from build123d import *

# Parameters (mm, degrees)
SKETCH_1_W          = 12
SKETCH_1_H          = 12
EXTRUDE_1_DEPTH     = 9.5
SKETCH_2_R          = 5.5
EXTRUDE_2_DEPTH     = 455
SKETCH_3_W          = 12
SKETCH_3_H          = 12
EXTRUDE_3_DEPTH     = 12.5
SKETCH_4_R          = 4
EXTRUDE_4_DEPTH     = 8
CUT_EXTRUDE_START   = -6
SKETCH_6_R          = 2.5
CUT_EXTRUDE_2_DEPTH = 6
FILLET_1_R          = 2
SKETCH_7_R          = 4
EXTRUDE_5_DEPTH     = 8


with BuildPart() as part:
    # 草图1 → 凸台-拉伸1 (new body)
    with BuildSketch(Plane.XY):
        Rectangle(SKETCH_1_W, SKETCH_1_H)
    extrude(amount=EXTRUDE_1_DEPTH)

    # 草图2 → 凸台-拉伸2 (add)
    with BuildSketch(Plane.XY.offset(9.5)):
        Circle(SKETCH_2_R)
    extrude(amount=EXTRUDE_2_DEPTH)

    # 草图3 → 凸台-拉伸3 (add)
    with BuildSketch(Plane.XY.offset(464.5)):
        Rectangle(SKETCH_3_W, SKETCH_3_H)
    extrude(amount=EXTRUDE_3_DEPTH)

    # 草图4 → 凸台-拉伸4 (add)
    with BuildSketch(Plane.XY.offset(477)):
        Circle(SKETCH_4_R)
    extrude(amount=EXTRUDE_4_DEPTH)

    # 草图6 → 切除-拉伸2 (cut)
    with BuildSketch(Plane(origin=(0, 6, 0), x_dir=(1, 0, 0), z_dir=(0, 1, 0)).offset(CUT_EXTRUDE_START)):
        with Locations((0, -4.75)):
            Circle(SKETCH_6_R)
        with Locations((0, -469.25)):
            Circle(SKETCH_6_R)
    extrude(amount=CUT_EXTRUDE_2_DEPTH, mode=Mode.SUBTRACT)

    # 圆角1
    fillet_1_edges = [part.edges().sort_by_distance(p)[0] for p in [
        (6, -6, 470.75),
        (6, 6, 470.75),
        (-6, 6, 470.75),
        (-6, -6, 470.75),
        (6, -6, 4.75),
        (-6, -6, 4.75),
        (-6, 6, 4.75),
        (6, 6, 4.75),
    ]]
    fillet(fillet_1_edges, radius=FILLET_1_R)

    # 草图7 → 凸台-拉伸5 (add)
    with BuildSketch(Plane(origin=(0, 0, 0), x_dir=(-1, 0, 0), z_dir=(0, 0, -1))):
        Circle(SKETCH_7_R)
    extrude(amount=EXTRUDE_5_DEPTH)


solid = part.part
Input: part model. Units: mm. Frame: model coordinates. A direction names the side the tool comes from. Coordinates: 2 decimals unless noted, no trailing zeros. Loops run counter-clockwise (first coordinate to the right, second up) from the corner with the lowest first, then second, coordinate; pieces in that order, holes last.
Q1. Contact query for flat-ended pins moving along their axis: pin 1 (2 mm diameter, centred on x = -0.5, z = 427, fed in from +Y); pin 2 (1.5 mm diameter, centred on x = 1, z = 469, fed in from +Y); pin 3 (6 mm diameter, centred on y = -3, z = 370, fed in from +X). Output: stop coordinate, or through.
Q2. Draft query along Z for faces 1 (the face through (3.92, 1.42, 0)), 2 (the face through (-0.867, -3.905, 480.944)), 3 (the face through (-3, -5, 464.5)). Return one class per face: +Z half, -Z half, draft (parallel to the pull), parting line (faces both ways), or undercut.
Q3. Cut plane B-B (z = 225). Output: boundary loops of the cut face in (x, y).
Q4. Material intervals for line 1 (Z direction, x = 0, y = 1.8); line 2 (Z direction, x = 0, y = 4.25); line 3 (Z direction, x = 4.75, y = -5), sorted ascending.
Q5. Set-up query: faces 4 (the face through (6, 0, 471)), 5 (the face through (-1.19, -5.37, 233.82)), 6 (the face through (0.867, -3.905, -3.944)), 7 (the face through (3.92, 1.42, 477)). Return all of +Z, -Z, +X, -X, +Y, -Y with unobstructed straight access to the full face (end or side cutting, diameter ignored); none if empty.
Q6. Cut plane A-A (x = 0). Output: boundary loops of the cut face in (y, z), then the cut area to 3 significant figures.
Working result:
1. pin 1: stops at y = 5.5
1. pin 2: stops at y = 0
1. pin 3: stops at x = 5.5
2. face 1: -Z half
2. face 2: draft
2. face 3: undercut
3. outline: circle Ø11 at (0, 0)
4. line 1: z = -8 to 2.25, 7.25 to 466.75, 471.75 to 485
4. line 2: z = 0 to 2.25, 7.25 to 466.75, 471.75 to 477
4. line 3: z = 0 to 9.5, 464.5 to 477
5. face 4: +Z, -Z, +X, +Y, -Y
5. face 5: none
5. face 6: -Z
5. face 7: +Z
6. outline: (-6, 0) - (-4, 0) - (-4, -8) - (4, -8) - (4, 0) - (6, 0) - (6, 2.25) - (0, 2.25) - (0, 7.25) - (6, 7.25) - (6, 9.5) - (5.5, 9.5) - (5.5, 464.5) - (6, 464.5) - (6, 466.75) - (0, 466.75) - (0, 471.75) - (6, 471.75) - (6, 477) - (4, 477) - (4, 485) - (-4, 485) - (-4, 477) - (-6, 477) - (-6, 464.5) - (-5.5, 464.5) - (-5.5, 9.5) - (-6, 9.5) - close
6. area: 5,340 mm2
